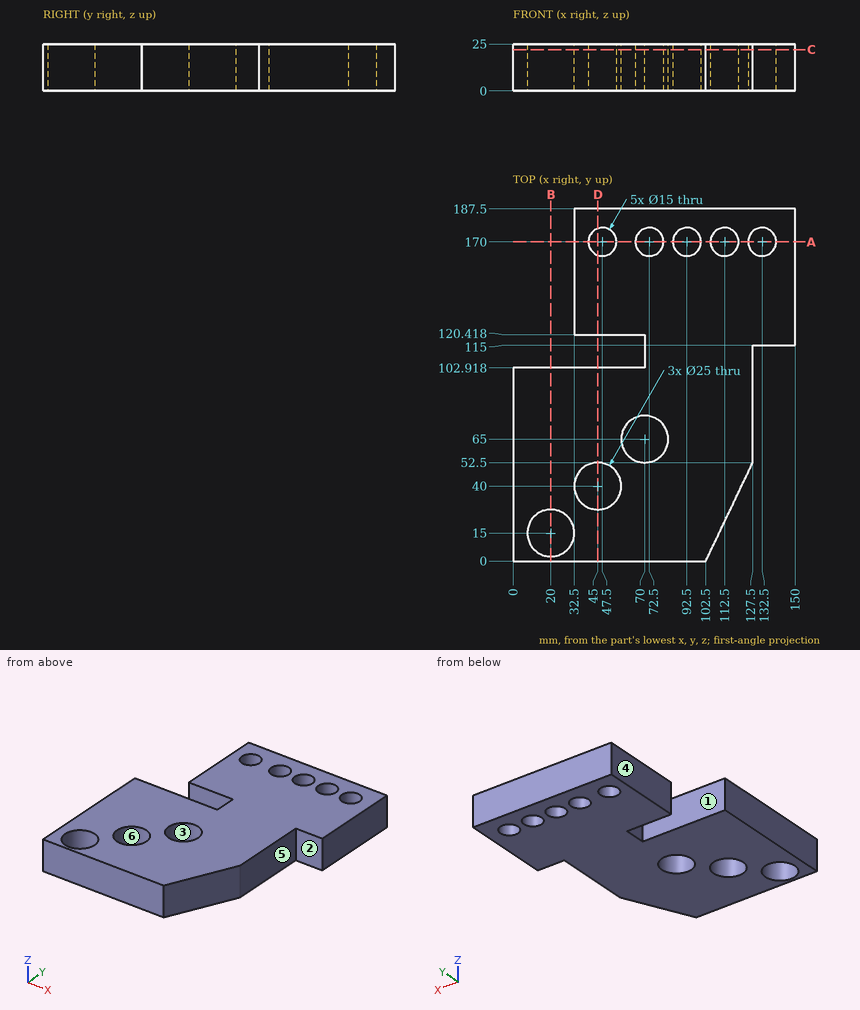
Part print with two shaded views. Sizes in mm from the minimum x, y, z corner. A direction names the side the tool comes from. Coordinates: 2 decimals unless noted, no trailing zeros. Order: outer loops, then holes, each group sorted by start corner. A loop starts at its lowest first (then second) coordinate and runs counter-clockwise, first axis right, second up. Notation, with made-up numbers: (58, -40) - (70, -40) arc R13 cw to (70, -27) - close; hole circle Ø6 at (87.25, 66.25). An arc over 180 degrees is marked (long way). Write item = value, one per line. Start each with the question number.
1) Saw through at B-B on x = 20. Write the cut outline in (y, z), then the cut area to 3 significant figures.
2) Wall check: line 1 along Y through (x, z) = (45, 5.25); line 2 along Y through (x, z) = (72.5, 15); line 3 along Y through (x, z) = (62.5, 2). Give the ranges that are in metal, low to high. Write a range as from..to.
3) Two-plate mould, pull along X, no slides. Class the marked faces 4, 5 and 6: pulls with the +X half, pulls with the -X half, needs draft (parallel to the pull), parting line crosses it, or undercut.
4) Saw through at C-C on z = 22. Count the separate pieces of the cut face and the enclosed holes in it, then the cut area to 3 significant figures.
5) Flat gauge pins, fed straight in: pin 1 Ø14 at (y, z) = (110.5, 13) entering from -X; pin 2 Ø12 at (x, y) = (47.5, 170) entering from -Z; pin 3 Ø8 at (x, z) = (21.5, 16.5) entering from +Y; pin 4 Ø1.5 at (y, z) = (168.5, 10) entering from -X. Where does each tip first touch, or does it go through?
6) 3-axis set-ups, long thin cutter, end or side, ignore diameter. For the marked faces 1, 2 and 3: which of +Z, -Z, +X, -X, +Y, -Y reach the whole face in a straight line?
7) Saw through at D-D on x = 45. Write the cut outline in (y, z).
8) Saw through at A-A on y = 170. Write the cut outline in (x, z), then the cut area to 3 significant figures.
From the geometry:
q1.outline = (0, 0) - (2.5, 0) - (2.5, 25) - (0, 25) - close; (27.5, 0) - (102.92, 0) - (102.92, 25) - (27.5, 25) - close
q1.area = 1,950 mm^2
q2.line_1 = 0..27.5, 52.5..102.92, 120.42..162.93, 177.07..187.5
q2.line_2 = 0..52.75, 77.25..162.5, 177.5..187.5
q2.line_3 = 0..55, 75..102.92, 120.42..187.5
q3.face_4 = pulls with the -X half
q3.face_5 = pulls with the +X half
q3.face_6 = undercut
q4.separate_pieces = 1
q4.enclosed_holes = 8
q4.area = 19,100 mm^2
q5.pin_1 = 70
q5.pin_2 = through
q5.pin_3 = 102.92
q5.pin_4 = 32.5
q6.face_1 = +Z, -Z, -X
q6.face_2 = +Z, -Z, +X, -Y
q6.face_3 = +Z, -Z
q7.outline = (0, 0) - (27.5, 0) - (27.5, 25) - (0, 25) - close; (52.5, 0) - (102.92, 0) - (102.92, 25) - (52.5, 25) - close; (120.42, 0) - (162.93, 0) - (162.93, 25) - (120.42, 25) - close; (177.07, 0) - (187.5, 0) - (187.5, 25) - (177.07, 25) - close
q8.outline = (32.5, 0) - (40, 0) - (40, 25) - (32.5, 25) - close; (55, 0) - (65, 0) - (65, 25) - (55, 25) - close; (80, 0) - (85, 0) - (85, 25) - (80, 25) - close; (100, 0) - (105, 0) - (105, 25) - (100, 25) - close; (120, 0) - (125, 0) - (125, 25) - (120, 25) - close; (140, 0) - (150, 0) - (150, 25) - (140, 25) - close
q8.area = 1,060 mm^2
